Check sheet for the modelled part. Datum: model origin and axes. Units: mm. A direction names the side the tool comes from. Round coordinates to 2 decimals unless told otherwise and drop trailing zeros. Order: outer loops, then holes, each group sorted by start corner. A loop starts at its lowest first (then second) coordinate and runs counter-clockwise, first axis right, second up.
(1) Tool access check on faces 1 (the cylindrical face through (-72.842, 0.089, 20.017)), 2 (the cylindrical face through (73.108, 0.089, 20.017)), 3 (the cylindrical face through (-17.88, -80.54, 12.86)), 4 (the flat face through (0, 63.45, 18)). Record the directions out of +Z, -Z, +X, -X, +Y, -Y that give a thin tool (end or side, any length) a straight path to the whole face; none if there is none.
(2) Depth check by flat-ended pin: pin 1 (1.5 mm diameter, centred on y = -22, z = 15, fed in from +X); pin 2 (2.5 mm diameter, centred on y = 0, z = 18, fed in from +X); pin 3 (5.5 mm diameter, centred on y = 0, z = 18, fed in from -X). Enter the tip coordinate at first touch or a pass-through.
(3) Thickness scan on probe 1 along Y at (x, z) = (0, 12.75); probe 2 along Z at (x, y) = (0, -75); probe 3 along Y at (x, z) = (15.5, 12). Record the ranges inside material, lowest first.
(4) Sectioned sample at C-C, the plane z = 18. Enter the section's corners in (x, y).
(5) Sectioned sample at D-D, the plane x = 70.5. Enter the section's corners in (y, z), and give its area (3 significant figures).
(6) Mould release check, pull along Z, two halves, no side actions. Record for faces 5 (the flat face through (-44, 70, 3)), 6 (the flat face through (-1, 1, 0)), 7 (the flat face through (-63.45, 0, 18)), 8 (the cylindrical face through (-67.453, -51.721, 1.479)): released by +Z, released by -Z, zero draft, split by the parting line, or undercut.
(7) Sectioned sample at A-A, the plane y = 0. Enter the section's corners in (x, z).
```python
from build123d import *

# Parameters (mm, degrees)
SKETCH1_R           = 85
BOSS_EXTRUDE2_DEPTH = 3
SKETCH2_R           = 82.5
BOSS_EXTRUDE3_DEPTH = 20
SKETCH3_R           = 50
CUT_EXTRUDE1_DEPTH  = 20
SKETCH9_R           = 2.0193
CUT_EXTRUDE5_DEPTH  = 19.05
CUT_EXTRUDE6_START  = 19.05
SKETCH10_R          = 2.0193
CUT_EXTRUDE6_DEPTH  = 19.05
SKETCH11_R          = 2.0193
CUT_EXTRUDE7_DEPTH  = 19.05
CUT_EXTRUDE8_START  = 19.05
SKETCH12_R          = 2.0193
CUT_EXTRUDE8_DEPTH  = 19.05


with BuildPart() as part:
    # Sketch1 → Boss-Extrude2 (new body)
    with BuildSketch(Plane.XY):
        Circle(SKETCH1_R)
    extrude(amount=BOSS_EXTRUDE2_DEPTH)

    # Sketch2 → Boss-Extrude3 (add)
    with BuildSketch(Plane.XY.offset(3)):
        Circle(SKETCH2_R)
    extrude(amount=BOSS_EXTRUDE3_DEPTH)

    # Sketch3 → Cut-Extrude1 (cut)
    with BuildSketch(Plane.XY.offset(23)):
        Circle(SKETCH3_R)
    extrude(amount=-CUT_EXTRUDE1_DEPTH, mode=Mode.SUBTRACT)

    # Sketch9 → Cut-Extrude5 (cut)
    with BuildSketch(Plane(origin=(0, 82.5, 0), x_dir=(-1, 0, 0), z_dir=(0, -1, 0))):
        with Locations((0, -18)):
            Circle(SKETCH9_R)
    extrude(amount=CUT_EXTRUDE5_DEPTH, mode=Mode.SUBTRACT)

    # Sketch10 → Cut-Extrude6 (cut)
    with BuildSketch(Plane(origin=(0, -82.5, 0), x_dir=(1, 0, 0), z_dir=(0, 1, 0)).offset(CUT_EXTRUDE6_START)):
        with Locations(Location((0, -18, 0), (0, 0, 180))):
            Circle(SKETCH10_R)
    extrude(amount=-CUT_EXTRUDE6_DEPTH, mode=Mode.SUBTRACT)

    # Sketch11 → Cut-Extrude7 (cut)
    with BuildSketch(Plane(origin=(82.5, 0, 0), x_dir=(0, 0, -1), z_dir=(1, 0, 0))):
        with Locations((-18, 0)):
            Circle(SKETCH11_R)
    extrude(amount=-CUT_EXTRUDE7_DEPTH, mode=Mode.SUBTRACT)

    # Sketch12 → Cut-Extrude8 (cut)
    with BuildSketch(Plane(origin=(-82.5, 0, 0), x_dir=(0, 0, -1), z_dir=(1, 0, 0)).offset(CUT_EXTRUDE8_START)):
        with Locations((-18, 0)):
            Circle(SKETCH12_R)
    extrude(amount=-CUT_EXTRUDE8_DEPTH, mode=Mode.SUBTRACT)


solid = part.part
```
Derived:
1. face 1: -X
1. face 2: +X
1. face 3: +Z
1. face 4: +Y
2. pin 1: stops at x = 79.72
2. pin 2: stops at x = 63.45
2. pin 3: stops at x = -82.5
3. probe 1: y = -82.5 to -50, 50 to 82.5
3. probe 2: z = 0 to 15.98, 20.02 to 23
3. probe 3: y = -81.03 to -47.54, 47.54 to 81.03
4. outline: (-82.48, -2.02) arc R82.5 ccw to (-2.02, -82.48) - (-2.02, -63.45) - (2.02, -63.45) - (2.02, -82.48) arc R82.5 ccw to (82.48, -2.02) - (63.45, -2.02) - (63.45, 2.02) - (82.48, 2.02) arc R82.5 ccw to (2.02, 82.48) - (2.02, 63.45) - (-2.02, 63.45) - (-2.02, 82.48) arc R82.5 ccw to (-82.48, 2.02) - (-63.45, 2.02) - (-63.45, -2.02) - close; hole circle Ø100 at (0, 0)
5. outline: (-47.48, 0) - (47.48, 0) - (47.48, 3) - (42.85, 3) - (42.85, 23) - (-42.85, 23) - (-42.85, 3) - (-47.48, 3) - close; hole circle Ø4.04 at (0, 18)
5. area: 1,990 mm2
6. face 5: released by +Z
6. face 6: released by -Z
6. face 7: undercut
6. face 8: zero draft
7. outline: (-85, 0) - (85, 0) - (85, 3) - (82.5, 3) - (82.5, 15.98) - (63.45, 15.98) - (63.45, 20.02) - (82.5, 20.02) - (82.5, 23) - (50, 23) - (50, 3) - (-50, 3) - (-50, 23) - (-82.5, 23) - (-82.5, 20.02) - (-63.45, 20.02) - (-63.45, 15.98) - (-82.5, 15.98) - (-82.5, 3) - (-85, 3) - close
